The drawing under review shows one solid part. Ordinate dimensions are in mm from its lowest x, y, z. A direction names the side the tool comes from. Give positions to 0.01 mm unless a question says otherwise; leave off trailing zeros. Write each loop counter-clockwise with the first axis right and the second up, starting at its lowest first coordinate (ties: lowest second). Pieces come first, ordered by that corner, then holes. Notation, with made-up numbers: M 85.5,53 L 141.5,53 A27 ccw 141.5,75 Z; hole C -31,-16 d10. An arc over 180 degrees is marked long. One line per item, written item: value. Start each with the question number.
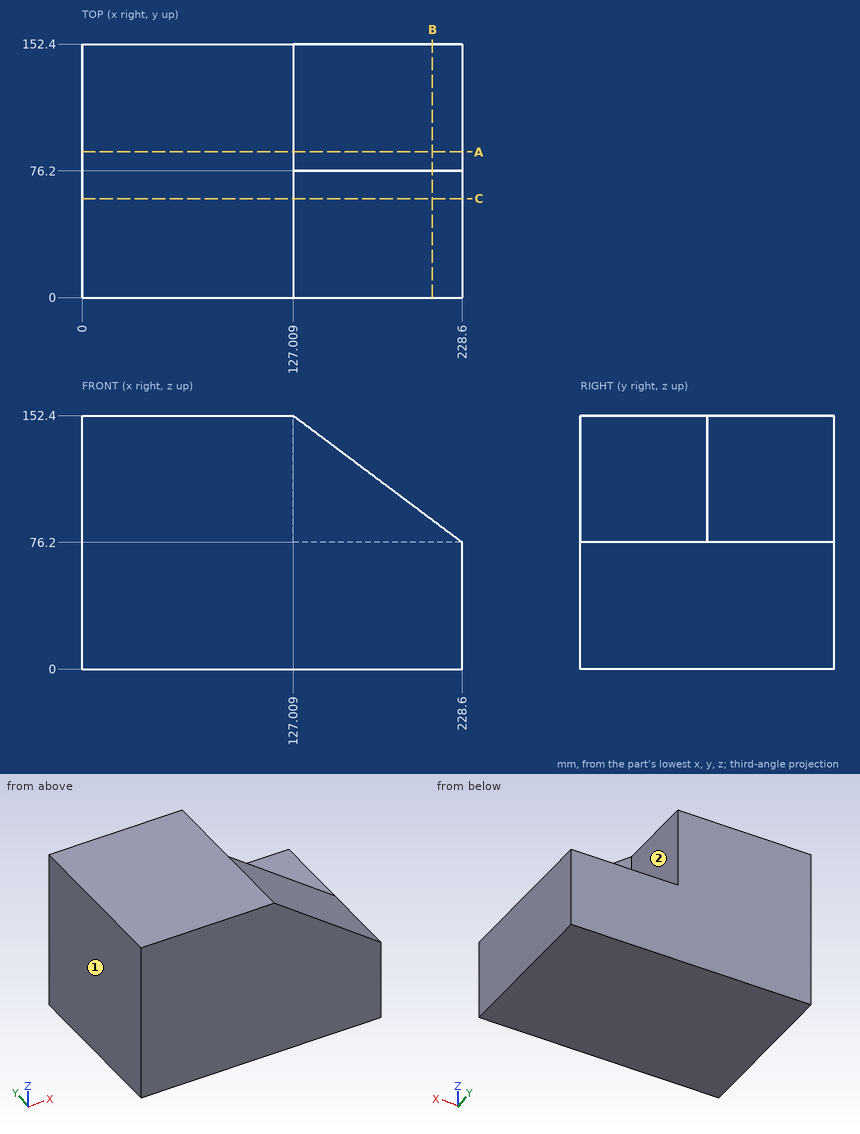
Q1. Machinability: for the marked faces 1 and 2, which of the approach directions +Z, -Z, +X, -X, +Y, -Y give a long, thin tool a straight path to every point of the face, cutting with its end or side? Answer none if there is none.
Q2. Take a section at B-B, the plane x = 210.5. Give the boundary of the cut face in (y, z).
Q3. Take a section at A-A, the plane y = 87.5. Give the boundary of the cut face in (x, z), then the cut area to 3 significant figures.
Q4. For P1, Ø4, axis at x = 164.5, y = 21.5, coming from the +Z side; P2, Ø1.5, axis at x = 154, z = 109, coming from the +Y side; P3, Ø5, axis at y = 61, z = 100, coming from the -X side; P4, Ø8, axis at x = 166, y = 69.5, coming from the +Z side (1 decimal), all flat-tipped, find the tip position at first contact; note any pin that passes through.
Q5. Take a section at C-C, the plane y = 59.5. Give the boundary of the cut face in (x, z).
Q6. Wall thickness on line 1 (X direction, y = 139, z = 125); line 2 (Y direction, x = 134, z = 130): over which ranges is each line inside the solid? List them lowest first. Write a range as from..to.
Results list:
1. face 1: +Z, -Z, -X, +Y, -Y
1. face 2: +Z, +X, +Y
2. outline: M 0,0 L 152.4,0 L 152.4,76.2 L 76.2,76.2 L 76.2,89.78 L 0,89.78 Z
3. outline: M 0,0 L 228.6,0 L 228.6,76.2 L 127.01,76.2 L 127.01,152.4 L 0,152.4 Z
3. area: 27,100 mm^2
4. P1: stops at z = 125.78
4. P2: stops at y = 76.2
4. P3: stops at x = 0
4. P4: stops at z = 126.2
5. outline: M 0,0 L 228.6,0 L 228.6,76.2 L 127.01,152.4 L 0,152.4 Z
6. line 1: x = 0..127.01
6. line 2: y = 0..76.2
